Source: three-view drawing plus pictorial views. Frame: mm from the lowest corner of the part. Coordinates: 2 decimals unless noted, no trailing zeros. Write each loop counter-clockwise with the first axis right and the second up, starting at its lowest first coordinate (ties: lowest second). Pieces come first, ordered by that corner, then holes. Notation, with made-up numbers: (58, 54.5) - (106, 54.5) arc R5 cw to (106, 60.5) - close; hole circle Ø8 at (-8, -6.5). An arc over 180 degrees is marked (long way). Put each result on its own line as item: value. Start each with the question number.
1. Line query: line 1 (Y direction, x = 55, z = 2.4); line 2 (X direction, y = 5.5, z = 3.2); line 3 (X direction, y = 23, z = 3.25). Output: solid intervals per line, ascending.
2. Cut plane C-C, the plane y = 15. Return loops of the section in (x, z), and give its area (4 significant figures).
3. Cut plane B-B, the plane y = 25. Return loops of the section in (x, z), and give its area (3 significant figures).
4. Cut plane D-D, the plane x = 30. Return loops of the section in (y, z), and give its area (4 significant figures).
5. Cut plane A-A, the plane x = 5. Return loops of the section in (y, z).
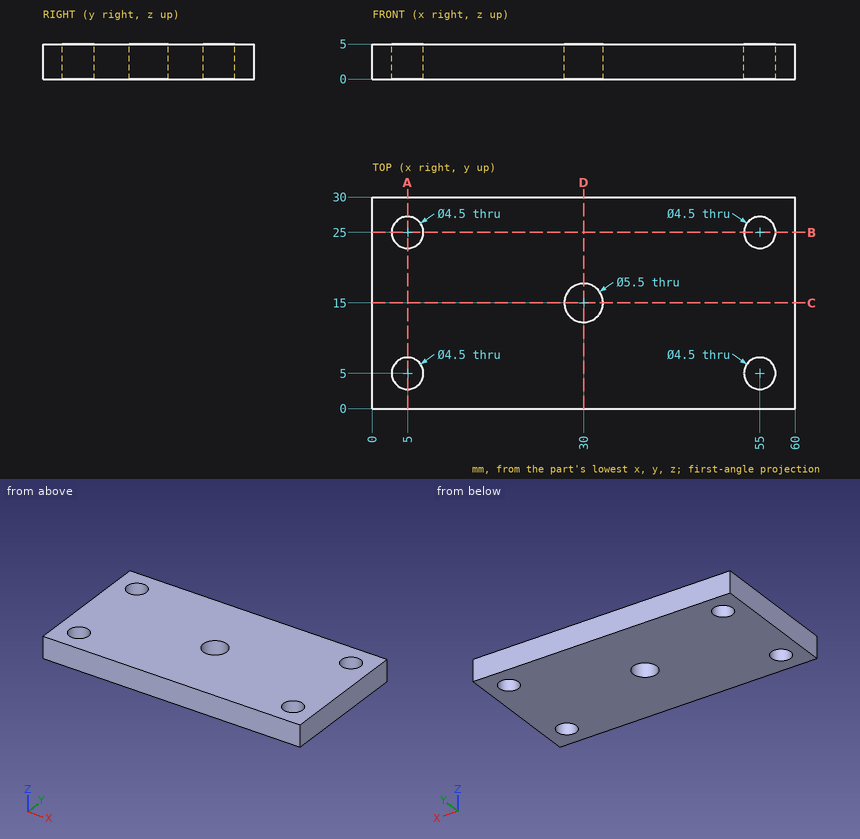
Report:
1. line 1: y = 0 to 2.75, 7.25 to 22.75, 27.25 to 30
1. line 2: x = 0 to 2.81, 7.19 to 52.81, 57.19 to 60
1. line 3: x = 0 to 3.97, 6.03 to 53.97, 56.03 to 60
2. outline: (0, 0) - (27.25, 0) - (27.25, 5) - (0, 5) - close; (32.75, 0) - (60, 0) - (60, 5) - (32.75, 5) - close
2. area: 272.5 mm^2
3. outline: (0, 0) - (2.75, 0) - (2.75, 5) - (0, 5) - close; (7.25, 0) - (52.75, 0) - (52.75, 5) - (7.25, 5) - close; (57.25, 0) - (60, 0) - (60, 5) - (57.25, 5) - close
3. area: 255 mm^2
4. outline: (0, 0) - (12.25, 0) - (12.25, 5) - (0, 5) - close; (17.75, 0) - (30, 0) - (30, 5) - (17.75, 5) - close
4. area: 122.5 mm^2
5. outline: (0, 0) - (2.75, 0) - (2.75, 5) - (0, 5) - close; (7.25, 0) - (22.75, 0) - (22.75, 5) - (7.25, 5) - close; (27.25, 0) - (30, 0) - (30, 5) - (27.25, 5) - close
